Read the model definition and answer for the solid it produces. Units are mm, in the model's axes. Face numbers are marked on the shaded views. A direction names the side the tool comes from. Coordinates: 2 decimals unless noted, no trailing zeros. Order: outer loops, then holes, each group sorted by start corner. A loop starts at its lowest first (then second) coordinate and runs counter-clockwise, first axis right, second up.
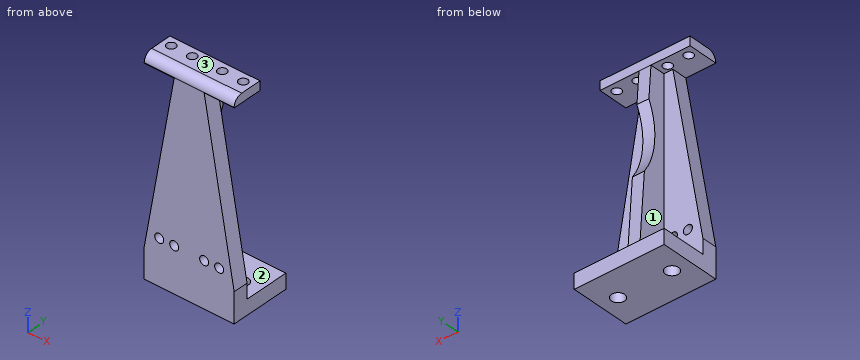
```python
from build123d import *

# Parameters (mm, degrees)
SKETCH_W     = 30
SKETCH_H     = 20
SKETCH_R     = 2.2
PAD_DEPTH    = 5
SKETCH001_R  = 1.5
PAD001_DEPTH = 5
SKETCH002_W  = 30
SKETCH002_H  = 10
SKETCH002_R  = 1.5
PAD002_DEPTH = 3
PAD003_DEPTH = 2
FILLET_R     = 2.9


with BuildPart() as part:
    # Sketch → Pad (new body)
    with BuildSketch(Plane.XY):
        with Locations((15, 10)):
            Rectangle(SKETCH_W, SKETCH_H)
        with Locations((6, 10)):
            Circle(SKETCH_R, mode=Mode.SUBTRACT)
        with Locations((24, 10)):
            Circle(SKETCH_R, mode=Mode.SUBTRACT)
    extrude(amount=PAD_DEPTH)

    # Sketch001 → Pad001 (join)
    with BuildSketch(Plane.XZ):
        Polygon((0, 0), (0, 10), (10, 67), (20, 67), (30, 10), (30, 0), align=None)
        with Locations((5, 15)):
            Circle(SKETCH001_R, mode=Mode.SUBTRACT)
        with Locations((10, 15)):
            Circle(SKETCH001_R, mode=Mode.SUBTRACT)
        with Locations((20, 15)):
            Circle(SKETCH001_R, mode=Mode.SUBTRACT)
        with Locations((25, 15)):
            Circle(SKETCH001_R, mode=Mode.SUBTRACT)
    extrude(amount=-PAD001_DEPTH)

    # Sketch002 → Pad002 (join)
    with BuildSketch(Plane.XY.offset(67)):
        with Locations((15, 5)):
            Rectangle(SKETCH002_W, SKETCH002_H)
        with Locations((3, 7)):
            Circle(SKETCH002_R, mode=Mode.SUBTRACT)
        with Locations((10, 7)):
            Circle(SKETCH002_R, mode=Mode.SUBTRACT)
        with Locations((20, 7)):
            Circle(SKETCH002_R, mode=Mode.SUBTRACT)
        with Locations((27, 7)):
            Circle(SKETCH002_R, mode=Mode.SUBTRACT)
    extrude(amount=PAD002_DEPTH)

    # Sketch003 → Pad003 (join, symmetric)
    with BuildSketch(Plane.YZ.offset(15)):
        with BuildLine():
            Line((0, 0), (15, 0))
            Line((15, 0), (12.551586, 32.808745))
            ThreePointArc((10.80907, 56.158468), (8.565166, 44.251132), (12.551586, 32.808745))
            Line((10.80907, 56.158468), (10, 67))
            Line((10, 67), (0, 67))
            Line((0, 67), (0, 0))
        make_face()
    extrude(amount=PAD003_DEPTH, both=True)

    # Fillet
    fillet_edges = [part.edges().sort_by_distance(p)[0] for p in [
        (15, 0, 70),
    ]]
    fillet(fillet_edges, radius=FILLET_R)


solid = part.part
```
1) Straight lines are drawn through the part: line 1 (Y direction, x = 21.75, z = 25); line 2 (Y direction, x = 3, z = 67.7). For each, find the intervals that lie inside material, in ascending order.
A:
line 1: y = 0 to 5
line 2: y = 0.06 to 5.5, 8.5 to 10
2) A cutting plane is placed at A-A, the plane y = 7. Determine the outline of the cut face in (x, z).
A:
outline: (0, 0) - (30, 0) - (30, 5) - (17, 5) - (17, 67) - (18.5, 67) - (18.5, 70) - (11.5, 70) - (11.5, 67) - (13, 67) - (13, 5) - (0, 5) - close; (0, 67) - (1.5, 67) - (1.5, 70) - (0, 70) - close; (4.5, 67) - (8.5, 67) - (8.5, 70) - (4.5, 70) - close; (21.5, 67) - (25.5, 67) - (25.5, 70) - (21.5, 70) - close; (28.5, 67) - (30, 67) - (30, 70) - (28.5, 70) - close
3) Which of the six approach directions +Z, -Z, +X, -X, +Y, -Y give full straight-line access (tool end or side, diameter ignored) to the marked faces 1, 2 and 3?
A:
face 1: -X, +Y
face 2: +Y
face 3: +Z, +X, -X, +Y, -Y
4) A cutting plane is placed at C-C, the plane z = 15. Determine the outline of the cut face in (x, y).
A:
outline: (0.88, 0) - (3.5, 0) - (3.5, 5) - (0.88, 5) - close; (6.5, 0) - (8.5, 0) - (8.5, 5) - (6.5, 5) - close; (11.5, 0) - (18.5, 0) - (18.5, 5) - (17, 5) - (17, 13.88) - (13, 13.88) - (13, 5) - (11.5, 5) - close; (21.5, 0) - (23.5, 0) - (23.5, 5) - (21.5, 5) - close; (26.5, 0) - (29.12, 0) - (29.12, 5) - (26.5, 5) - close
5) A cutting plane is placed at D-D, the plane y = 11.5. Determine the outline of the cut face in (x, z).
A:
outline: (0, 0) - (4.39, 0) - (4.39, 5) - (0, 5) - close; (7.61, 0) - (22.39, 0) - (22.39, 5) - (17, 5) - (17, 34.51) - (13, 34.51) - (13, 5) - (7.61, 5) - close; (25.61, 0) - (30, 0) - (30, 5) - (25.61, 5) - close
6) A cutting plane is placed at B-B, the plane x = 15.25. Determine the outline of the cut face in (y, z), and give its area (3 significant figures).
A:
outline: (0, 0) - (20, 0) - (20, 5) - (14.63, 5) - (12.55, 32.81) arc R23.5 cw to (10.81, 56.16) - (10, 67) - (10, 70) - (2.9, 70) arc R2.9 ccw to (0, 67.1) - close
area: 842 mm2
7) Flat-ended cylindrical pins translate along their axes: pin 1 Ø3.5 at (x, y) = (6, 10) entering from -Z; pin 2 Ø2.5 at (x, y) = (27, 7) entering from +Z; pin 3 Ø12 at (y, z) = (5, 35) entering from +X. Find the tip coordinate at first contact, or state that the pin passes through.
A:
pin 1: stops at z = 67
pin 2: stops at z = 5
pin 3: stops at x = 26.67
